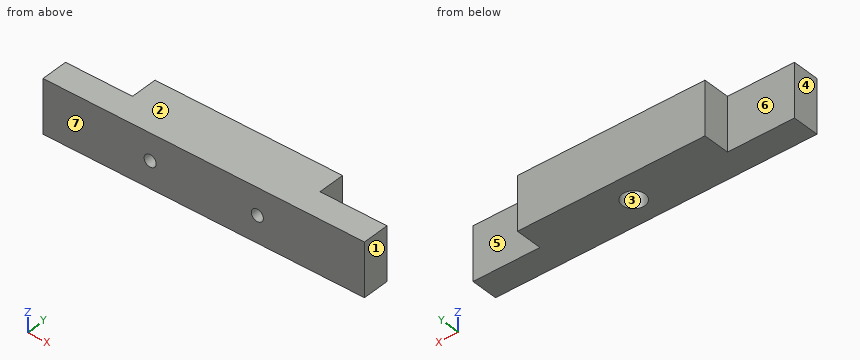
```python
from build123d import *

# Parameters (mm, degrees)
SKETCH1_W           = 120
SKETCH1_H           = 20
BOSS_EXTRUDE1_DEPTH = 20
SKETCH2_W           = 25
SKETCH2_H           = 10
CUT_EXTRUDE1_DEPTH  = 20
SKETCH5_R           = 4.25
CUT_EXTRUDE3_DEPTH  = 10
SKETCH6_R           = 2.25
CUT_EXTRUDE4_DEPTH  = 10


with BuildPart() as part:
    # Sketch1 → Boss-Extrude1 (new body)
    with BuildSketch(Plane(origin=(0, 0, 0), x_dir=(1, 0, 0), z_dir=(0, 1, 0))):
        with Locations((60, 10)):
            Rectangle(SKETCH1_W, SKETCH1_H)
    extrude(amount=BOSS_EXTRUDE1_DEPTH)

    # Sketch2 → Cut-Extrude1 (cut)
    with BuildSketch(Plane.XY):
        with Locations((12.5, 15)):
            Rectangle(SKETCH2_W, SKETCH2_H)
        with Locations((107.5, 15)):
            Rectangle(SKETCH2_W, SKETCH2_H)
    extrude(amount=-CUT_EXTRUDE1_DEPTH, mode=Mode.SUBTRACT)

    # Sketch5 → Cut-Extrude3 (cut)
    with BuildSketch(Plane(origin=(0, 0, -20), x_dir=(-1, 0, 0), z_dir=(0, 0, -1))):
        with Locations((-60, 10)):
            Circle(SKETCH5_R)
    extrude(amount=-CUT_EXTRUDE3_DEPTH, mode=Mode.SUBTRACT)

    # Sketch6 → Cut-Extrude4 (cut)
    with BuildSketch(Plane(origin=(0, 0, 0), x_dir=(-1, 0, 0), z_dir=(0, -1, 0))):
        with Locations(Location((-80, 10, 0), (0, 0, 90))):
            Circle(SKETCH6_R)
        with Locations(Location((-40, 10, 0), (0, 0, 90))):
            Circle(SKETCH6_R)
    extrude(amount=-CUT_EXTRUDE4_DEPTH, mode=Mode.SUBTRACT)


solid = part.part
```
For this review, take the finished solid that the model builds, in its own axes (mm). Face numbers are marked on the shaded views. A direction names the side the tool comes from. Give positions to 0.01 mm unless a question says otherwise; leave off trailing zeros. Write each loop counter-clockwise with the first axis right and the second up, starting at its lowest first coordinate (ties: lowest second). Pieces come first, ordered by that corner, then holes. Notation, with made-up numbers: M 20,45 L 33,45 A21 ccw 33,72 Z; hole C 70.5,37.5 d6. An arc over 180 degrees is marked long. One line per item, written item: value.
1) Take a section at D-D, the plane y = 8.75. Write out the cut boundary in (x, z), then the cut area to 3 significant figures.
Results are:
outline: M 0,-20 L 55.94,-20 L 55.94,-10 L 64.06,-10 L 64.06,-20 L 120,-20 L 120,0 L 0,0 Z; hole C 40,-10 d4.5; hole C 80,-10 d4.5
area: 2,290 mm²
2) For line 1 (X direction, y = 3.25, z = -10); line 2 (X direction, y = 8.75, z = -8.5); line 3 (Y direction, x = 60, z = -16.5), list the stretches that pass through material, from the lowest coordinate up. Write a range as from..to.
Results are:
line 1: x = 0..37.75, 42.25..77.75, 82.25..120
line 2: x = 0..38.32, 41.68..78.32, 81.68..120
line 3: y = 0..5.75, 14.25..20
3) Take a section at B-B, the plane z = -2.25. Write out the cut boundary in (x, y), then the cut area to 3 significant figures.
Results are:
outline: M 0,0 L 120,0 L 120,10 L 95,10 L 95,20 L 25,20 L 25,10 L 0,10 Z
area: 1,900 mm²
4) Take a section at A-A, the plane x = 60. Write out the cut boundary in (y, z), then the cut area to 3 significant figures.
Results are:
outline: M 0,-20 L 5.75,-20 L 5.75,-10 L 14.25,-10 L 14.25,-20 L 20,-20 L 20,0 L 0,0 Z
area: 315 mm²
5) For the marked faces 5, 6 and 7, list the 3-axis set-ups (+Z, -Z, +X, -X, +Y, -Y) from which the entire face can be reached by the end or side of a thin tool; tool diameter is ignored.
Results are:
face 5: +Z, -Z, +X, +Y
face 6: +Z, -Z, -X, +Y
face 7: +Z, -Z, +X, -X, -Y
6) For P1, Ø12, axis at y = 8.5, z = -2.5, coming from the -X side; P2, Ø7.5, axis at x = 60, y = 10, coming from the -Z side; P3, Ø11, axis at y = 16, z = -5.5, coming from the -X side; P4, Ø6, axis at y = 15, z = -7, coming from the +X side, all flat-tipped, find the tip position at first contact; note any pin that passes through.
Results are:
P1: stops at x = 0
P2: stops at z = -10
P3: stops at x = 25
P4: stops at x = 95
7) Take a section at C-C, the plane z = -16.25. Write out the cut boundary in (x, y).
Results are:
outline: M 0,0 L 120,0 L 120,10 L 95,10 L 95,20 L 25,20 L 25,10 L 0,10 Z; hole C 60,10 d8.5
8) The part is to be moulded in two halves that separate along X. For the marked faces 1, 2, 3 and 4, say which applies: +X half, -X half, draft (parallel to the pull), parting line (faces both ways), or undercut.
Results are:
face 1: +X half
face 2: draft
face 3: undercut
face 4: -X half
